Model file for the job. Use its own axes, mm. Give positions to 0.01 mm unless a question says otherwise; leave off trailing zeros. Write each loop counter-clockwise with the first axis right and the second up, starting at its lowest first coordinate (ties: lowest second). Pieces come first, ordered by that corner, then holes. Notation, with made-up numbers: (7, 81) - (22, 81) arc R14 cw to (22, 96) - close; hole circle Ø7 at (16, 29.25). An arc over 180 degrees is marked (long way). Use CSV: the item, a comma, the result in double quotes.
from build123d import *

# Parameters (mm, degrees)
F1_DEPTH = 7
F2_R     = 1.5


with BuildPart() as f1:
    # F0 (on Top) → F1 (new body)
    with BuildSketch(Plane.XY):
        with BuildLine():
            ThreePointArc((-5, -8.660254), (-5, 8.660254), (10, 0))
            ThreePointArc((10, 0), (8.660254, -5), (5, -8.660254))
            Line((5, -8.660254), (5, -15.198684))
            ThreePointArc((5, -15.198684), (12.961481, -9.380832), (16, 0))
            ThreePointArc((16, 0), (-9.380832, 12.961481), (-5, -15.198684))
            Line((-5, -15.198684), (-5, -8.660254))
        make_face()
    extrude(amount=F1_DEPTH)

    # F2
    f2_edges = [f1.edges().sort_by_distance(p)[0] for p in [
        (-5, -15.198684, 3.5),
        (5, -15.198684, 3.5),
    ]]
    fillet(f2_edges, radius=F2_R)


solid = f1.part
(1) Flat gauge pins, fed straight in: P1, Ø2, axis at y = -11.5, z = 5, coming from the +X side; P2, Ø4, axis at x = -4, z = 2.5, coming from the -Y side; P3, Ø3, axis at x = -5, z = 3, coming from the +Y side. Where does each tip first touch, or does it go through?
Checked values:
P1,"stops at x = 12.07"
P2,"stops at y = -14.38"
P3,"stops at y = 15.61"
(2) Saw through at D-D, the plane y = 14.5. List the corners of the cut face in (x, z), then the cut area to 3 significant figures.
Checked values:
outline,"(-6.76, 0) - (6.76, 0) - (6.76, 7) - (-6.76, 7) - close"
area,"94.7 mm^2"
(3) Saw through at C-C, the plane x = 0. List the corners of the cut face in (y, z), then the cut area to 3 significant figures.
Checked values:
outline,"(10, 0) - (16, 0) - (16, 7) - (10, 7) - close"
area,"42.0 mm^2"
(4) Saw through at A-A, the plane z = 6.25. List the corners of the cut face in (x, y).
Checked values:
outline,"(-7.17, -14.3) arc R1.5 ccw to (-5, -12.96) - (-5, -8.66) arc R10 cw (long way) to (5, -8.66) - (5, -12.96) arc R1.5 ccw to (7.17, -14.3) arc R16 ccw (long way) to start"
(5) Pull direction X, two halves, no side cores. Call faces 1 (the face through (-5, -11, 3)), 2 (the face through (0, 11, 0)), 3 (the face through (5, -11, 3)): released by +X, released by -X, zero draft, split by the parting line, or undercut.
Checked values:
face 1,"undercut"
face 2,"zero draft"
face 3,"undercut"
(6) Wall check: probe 1 along Y at (x, z) = (9, 5); probe 2 along Y at (x, z) = (0, 5.5); probe 3 along Y at (x, z) = (-5.5, 6.5). Give the ranges that are in metal, low to high. Write a range as [from, to].
Checked values:
probe 1,"y = [-13.23, -4.36], [4.36, 13.23]"
probe 2,"y = [10, 16]"
probe 3,"y = [-14.08, -8.35], [8.35, 15.02]"
(7) Saw through at B-B, the plane x = 8.5. List the corners of the cut face in (y, z), then the cut area to 3 significant figures.
Checked values:
outline,"(-13.56, 0) - (-5.27, 0) - (-5.27, 7) - (-13.56, 7) - close; (5.27, 0) - (13.56, 0) - (13.56, 7) - (5.27, 7) - close"
area,"116 mm^2"
